Autodesk Inventor part; units mm, degrees
ref_plane "YZ Plane" through (0, 0, 0) normal (1, 0, 0) x (0, 1, 0)
ref_plane "XZ Plane" through (0, 0, 0) normal (0, 1, 0) x (-1, 0, 0)
ref_plane "XY Plane" through (0, 0, 0) normal (0, 0, 1) x (1, 0, 0)
sketch "Náčrt1" plane through (0, 0, 0) normal (0, 0, 1) x (1, 0, 0)
  line L0 (-3, -1) -> (3, -1)
  line L1 (3, -1) -> (3, 1)
  line L2 (3, 1) -> (-3, 1)
  line L3 (-3, 1) -> (-3, -1)
  line L4 (-3, -1) -> (3, 1) construction
  line L5 (3, -1) -> (-3, 1) construction
  line L6 (3, 1) -> (1, 1)
  line L7 (1, 1) -> (1, -3.5)
  line L8 (1, -3.5) -> (3, -3.5)
  line L9 (3, -3.5) -> (3, 1)
  point P0 (0, 0)
  point P1 (1, -1)
  dimension "d0" = 6
  dimension "d1" = 2
  dimension "d2" = 2
  dimension "d3" = 4.5
extrude "Vysunutí1" add sketch "Náčrt1" along normal blind 3
chamfer "Zkosení1" distance 1.5 angle 45 1 edges at (-3, 1, 1.5)
properties part number "sonar-liner_3D tisk"
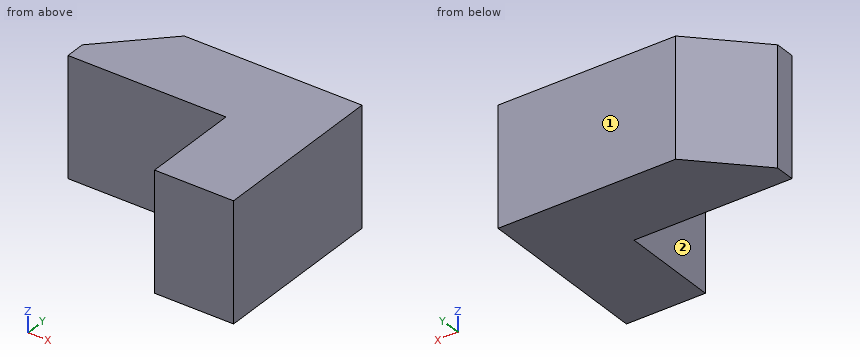
The listing builds one solid part. Answer for the finished solid, in the listing's coordinates (mm). Face numbers are marked on the shaded views. A direction names the side the tool comes from. Give positions to 0.01 mm unless a question says otherwise; leave off trailing zeros. Write each loop counter-clockwise with the first axis right and the second up, starting at its lowest first coordinate (ties: lowest second). Pieces come first, ordered by that corner, then holes.
Item 1: Section A-A, the plane z = 1.45 is taken. Write down the section's boundary in (x, y).
Item 2: Flat-ended cylindrical pins translate along their axes: P1, Ø1.2, axis at y = -2, z = 1, coming from the -X side; P2, Ø1.5, axis at x = -0.5, z = 1, coming from the -Y side. Find the tip coordinate at first contact, or state that the pin passes through.
Item 3: Section C-C, the plane y = -3 is taken. Write down the section's boundary in (x, z), plus the area to 3 significant figures.
Item 4: Find the intervals of material crossed by line 1 along Y through (x, z) = (-0.7, 1.7); line 2 along X through (y, z) = (-2.95, 2.5); line 3 along Y through (x, z) = (-1.65, 0.45), in increasing order.
Item 5: Section B-B, the plane x = -2.25 is taken. Write down the section's boundary in (y, z), plus the area to 3 significant figures.
Item 6: Which of the six approach directions +Z, -Z, +X, -X, +Y, -Y give full straight-line access (tool end or side, diameter ignored) to the marked faces 1 and 2?
Completed:
1. outline: (-3, -1) - (1, -1) - (1, -3.5) - (3, -3.5) - (3, 1) - (-1.5, 1) - (-3, -0.5) - close
2. P1: stops at x = 1
2. P2: stops at y = -1
3. outline: (1, 0) - (3, 0) - (3, 3) - (1, 3) - close
3. area: 6.00 mm2
4. line 1: y = -1 to 1
4. line 2: x = 1 to 3
4. line 3: y = -1 to 0.85
5. outline: (-1, 0) - (0.25, 0) - (0.25, 3) - (-1, 3) - close
5. area: 3.75 mm2
6. face 1: +Z, -Z, +X, -X, +Y
6. face 2: +Z, -Z, -X, -Y
